Geometry check sheet. Reference: the model listing, model coordinates, mm. Face numbers are marked on the shaded views. A direction names the side the tool comes from. Coordinates: 2 decimals unless noted, no trailing zeros. Write each loop counter-clockwise with the first axis right and the second up, starting at its lowest first coordinate (ties: lowest second). Pieces come first, ordered by that corner, then holes. Notation, with made-up numbers: (-22, 81.5) -> (-1, 81.5) arc R20 ccw to (-1, 119.5) -> close; hole circle Ø5 at (-7, 24). An arc over 180 degrees is marked (long way). Answer in a Markdown table with one row per item. Add a question column.
Q1. Section check A-A, the plane z = 7.5. Record the boundary of the cut face in (x, y) (3 decimals), and give its area (3 significant figures).
Q2. Section check C-C, the plane x = -22. Record the boundary of the cut face in (y, z) (3 decimals), and give its area (3 significant figures).
Q3. Section check B-B, the plane y = 52.5. Record the boundary of the cut face in (x, z) (3 decimals), and give its area (3 significant figures).
Q4. Release check for a two-part mould opening along X. For the marked faces 4, 5 and 6 record: pulls with the +X half, pulls with the -X half, needs draft (parallel to the pull), parting line crosses it, or undercut.
Q5. Tool access check on the marked faces 1, 2 and 3. Record the directions out of +Z, -Z, +X, -X, +Y, -Y that give a thin tool (end or side, any length) a straight path to the whole face; none if there is none.
Q6. Thickness scan on line 1 (Y direction, x = 88.9, z = -6); line 2 (Y direction, x = 88.9, z = 1); line 3 (X direction, y = 44.45, z = 8). Record the ranges inside material, lowest first.
Q7. Section check D-D, the plane y = 9.5. Record the boundary of the cut face in (x, z) (3 decimals), and give its area (3 significant figures).
Q8. Gauge pin test, flat ends, axial feed: P1, Ø3, axis at y = 25, z = 5, coming from the +X side; P2, Ø1.3, axis at y = 23.5, z = 6.5, coming from the -X side; P3, Ø11.5, axis at x = 53.5, y = 9, coming from the +Z side (3 decimals). Record the tip position at first contact, or that the pin passes through.
```python
from build123d import *

# Parameters (mm, degrees)
SKETCH1_W           = 215.9
SKETCH1_H           = 19.05
BOSS_EXTRUDE1_DEPTH = 88.9
SKETCH2_W           = 25.654
SKETCH2_H           = 88.9
CUT_EXTRUDE1_DEPTH  = 5.08
CUT_EXTRUDE2_DEPTH  = 6.35
CUT_EXTRUDE3_DEPTH  = 141.54029102
CUT_EXTRUDE4_DEPTH  = 10.922
CUT_EXTRUDE5_DEPTH  = 6.35
SKETCH9_R           = 3.3734375
SKETCH9_R_2         = 1.5875
CUT_EXTRUDE6_DEPTH  = 142.135803395
SKETCH10_R          = 4.7625
CUT_EXTRUDE7_DEPTH  = 6.35


with BuildPart() as part:
    # Sketch1 → Boss-Extrude1 (new body)
    with BuildSketch(Plane(origin=(0, 0, 0), x_dir=(1, 0, 0), z_dir=(0, 1, 0))):
        Rectangle(SKETCH1_W, SKETCH1_H)
    extrude(amount=BOSS_EXTRUDE1_DEPTH)

    # Sketch2 → Cut-Extrude1 (cut)
    with BuildSketch(Plane.XY.offset(9.525)):
        with Locations((50.673, 44.45)):
            Rectangle(SKETCH2_W, SKETCH2_H)
    extrude(amount=-CUT_EXTRUDE1_DEPTH, mode=Mode.SUBTRACT)

    # Sketch3 → Cut-Extrude2 (cut)
    with BuildSketch(Plane.XY.offset(9.525)):
        with BuildLine():
            Line((-57.15, 82.55), (25.4, 82.55))
            ThreePointArc((25.4, 82.55), (29.890128061, 80.690128061), (31.75, 76.2))
            Line((31.75, 76.2), (31.75, 12.7))
            ThreePointArc((31.75, 12.7), (29.890128061, 8.209871939), (25.4, 6.35))
            Line((25.4, 6.35), (-57.15, 6.35))
            ThreePointArc((-57.15, 6.35), (-61.640128061, 8.209871939), (-63.5, 12.7))
            Line((-63.5, 12.7), (-63.5, 76.2))
            ThreePointArc((-63.5, 76.2), (-61.640128061, 80.690128061), (-57.15, 82.55))
        make_face()
    extrude(amount=-CUT_EXTRUDE2_DEPTH, mode=Mode.SUBTRACT)

    # Sketch6 → Cut-Extrude3 (cut, through all)
    with BuildSketch(Plane.XY.offset(4.445)):
        with BuildLine():
            Line((46.736, 69.85), (54.61, 69.85))
            ThreePointArc((54.61, 69.85), (59.100128061, 67.990128061), (60.96, 63.5))
            Line((60.96, 63.5), (60.96, 25.4))
            ThreePointArc((60.96, 25.4), (59.100128061, 20.909871939), (54.61, 19.05))
            Line((54.61, 19.05), (46.736, 19.05))
            ThreePointArc((46.736, 19.05), (42.245871939, 20.909871939), (40.386, 25.4))
            Line((40.386, 25.4), (40.386, 63.5))
            ThreePointArc((40.386, 63.5), (42.245871939, 67.990128061), (46.736, 69.85))
        make_face()
    extrude(amount=-CUT_EXTRUDE3_DEPTH, mode=Mode.SUBTRACT)

    # Sketch5 → Cut-Extrude4 (cut)
    with BuildSketch(Plane.XY.offset(4.445)):
        with BuildLine():
            Line((44.196, 72.39), (57.15, 72.39))
            ThreePointArc((57.15, 72.39), (61.640128061, 70.530128061), (63.5, 66.04))
            Line((63.5, 66.04), (63.5, 22.86))
            ThreePointArc((63.5, 22.86), (61.640128061, 18.369871939), (57.15, 16.51))
            Line((57.15, 16.51), (44.196, 16.51))
            ThreePointArc((44.196, 16.51), (39.705871939, 18.369871939), (37.846, 22.86))
            Line((37.846, 22.86), (37.846, 66.04))
            ThreePointArc((37.846, 66.04), (39.705871939, 70.530128061), (44.196, 72.39))
        make_face()
    extrude(amount=-CUT_EXTRUDE4_DEPTH, mode=Mode.SUBTRACT)

    # Sketch8 → Cut-Extrude5 (cut)
    with BuildSketch(Plane.XY.offset(9.525)):
        with BuildLine():
            ThreePointArc((-98.298, 26.433896204), (-68.58, 44.45), (-98.298, 62.466103796))
            Line((-98.298, 62.466103796), (-98.298, 26.433896204))
        make_face()
        with BuildLine():
            Line((-98.298, 62.466103796), (-98.298, 66.675))
            ThreePointArc((-98.298, 66.675), (-101.125005348, 73.499994652), (-107.95, 76.327))
            Line((-107.95, 76.327), (-107.95, 12.573))
            ThreePointArc((-107.95, 12.573), (-101.125005348, 15.400005348), (-98.298, 22.225))
            Line((-98.298, 22.225), (-98.298, 26.433896204))
            Line((-98.298, 26.433896204), (-98.298, 62.466103796))
        make_face()
    cut_extrude5 = extrude(amount=-CUT_EXTRUDE5_DEPTH, mode=Mode.SUBTRACT)

    # Sketch9 → Cut-Extrude6 (cut, through all)
    with BuildSketch(Plane.XY.offset(9.525)):
        with Locations((-88.9, 44.45)):
            Circle(SKETCH9_R)
        with Locations((-88.9, 57.15)):
            Circle(SKETCH9_R_2)
    cut_extrude6 = extrude(amount=-CUT_EXTRUDE6_DEPTH, mode=Mode.SUBTRACT)

    # Sketch10 → Cut-Extrude7 (cut)
    with BuildSketch(Plane(origin=(0, 0, -9.525), x_dir=(-1, 0, 0), z_dir=(0, 0, -1))):
        with Locations((88.9, 44.45)):
            Circle(SKETCH10_R)
    cut_extrude7 = extrude(amount=-CUT_EXTRUDE7_DEPTH, mode=Mode.SUBTRACT)

    # Mirror1: Cut-Extrude5, Cut-Extrude6, Cut-Extrude7 across plane
    add(cut_extrude5.mirror(Plane(origin=(0, 0, 0), x_dir=(0, 0, 1), z_dir=(1, 0, 0))), mode=Mode.SUBTRACT)
    add(cut_extrude6.mirror(Plane(origin=(0, 0, 0), x_dir=(0, 0, 1), z_dir=(1, 0, 0))), mode=Mode.SUBTRACT)
    add(cut_extrude7.mirror(Plane(origin=(0, 0, 0), x_dir=(0, 0, 1), z_dir=(1, 0, 0))), mode=Mode.SUBTRACT)


solid = part.part
```
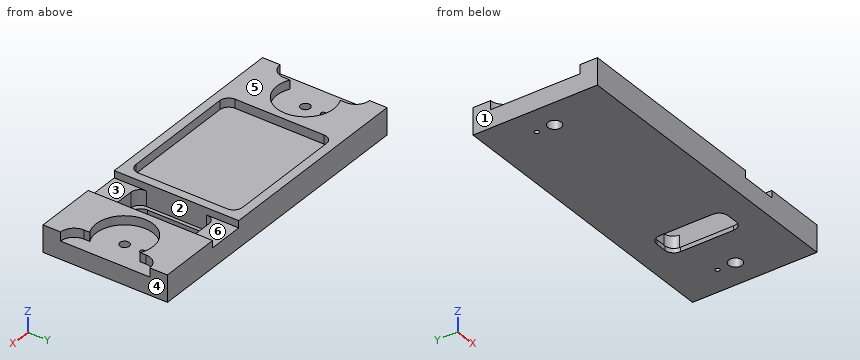
Calculated:
| question | item | result |
|---|---|---|
| 1 | outline | (-107.95, 0) -> (37.846, 0) -> (37.846, 88.9) -> (-107.95, 88.9) -> (-107.95, 76.327) arc R9.652 cw to (-98.298, 66.675) -> (-98.298, 62.466) arc R20.32 cw (long way) to (-98.298, 26.434) -> (-98.298, 22.225) arc R9.652 cw to (-107.95, 12.573) -> close; (63.5, 0) -> (107.95, 0) -> (107.95, 12.573) arc R9.652 cw to (98.298, 22.225) -> (98.298, 26.434) arc R20.32 cw (long way) to (98.298, 62.466) -> (98.298, 66.675) arc R9.652 cw to (107.95, 76.327) -> (107.95, 88.9) -> (63.5, 88.9) -> close; hole (-63.5, 12.7) arc R6.35 ccw to (-57.15, 6.35) -> (25.4, 6.35) arc R6.35 ccw to (31.75, 12.7) -> (31.75, 76.2) arc R6.35 ccw to (25.4, 82.55) -> (-57.15, 82.55) arc R6.35 ccw to (-63.5, 76.2) -> close |
| 1 | area | 6,510 mm² |
| 2 | outline | (0, -9.525) -> (88.9, -9.525) -> (88.9, 9.525) -> (82.55, 9.525) -> (82.55, 3.175) -> (6.35, 3.175) -> (6.35, 9.525) -> (0, 9.525) -> close |
| 2 | area | 1,210 mm² |
| 3 | outline | (-107.95, -9.525) -> (40.386, -9.525) -> (40.386, -6.477) -> (37.846, -6.477) -> (37.846, 9.525) -> (31.75, 9.525) -> (31.75, 3.175) -> (-63.5, 3.175) -> (-63.5, 9.525) -> (-70.243, 9.525) -> (-70.243, 3.175) -> (-107.95, 3.175) -> close; (60.96, -9.525) -> (107.95, -9.525) -> (107.95, 3.175) -> (70.243, 3.175) -> (70.243, 9.525) -> (63.5, 9.525) -> (63.5, -6.477) -> (60.96, -6.477) -> close |
| 3 | area | 2,560 mm² |
| 4 | face 4 | pulls with the +X half |
| 4 | face 5 | needs draft |
| 4 | face 6 | undercut |
| 5 | face 1 | +Z, -Z, -X, +Y, -Y |
| 5 | face 2 | +Z |
| 5 | face 3 | +Z, +Y, -Y |
| 6 | line 1 | y = 0 to 39.69, 49.21 to 55.56, 58.74 to 88.9 |
| 6 | line 2 | y = 0 to 41.08, 47.82 to 55.56, 58.74 to 88.9 |
| 6 | line 3 | x = -68.58 to -63.5, 31.75 to 37.85, 63.5 to 68.58 |
| 7 | outline | (-107.95, -9.525) -> (107.95, -9.525) -> (107.95, 9.525) -> (63.5, 9.525) -> (63.5, 4.445) -> (37.846, 4.445) -> (37.846, 9.525) -> (30.885, 9.525) -> (30.885, 3.175) -> (-62.635, 3.175) -> (-62.635, 9.525) -> (-107.95, 9.525) -> close |
| 7 | area | 3,390 mm² |
| 8 | P1 | stops at x = 98.3 |
| 8 | P2 | stops at x = -98.3 |
| 8 | P3 | stops at z = 4.445 |
